```python
from build123d import *

# Parameters (mm, degrees)
F2_R = 9
F3_R = 5


with BuildPart() as f1:
    # F0 (on Front) → F1 (revolve)
    with BuildSketch(Plane.XZ):
        with BuildLine():
            Line((0, 4.25), (0, 0))
            Line((0, 0), (64, 0))
            Line((64, 0), (64, 9))
            Line((64, 9), (20.85148, 9))
            ThreePointArc((20.85148, 9), (13.607068, 7.913606), (7, 4.75))
            Line((7, 4.75), (1.936492, 4.75))
            Line((1.936492, 4.75), (0, 4.25))
        make_face()
    revolve(axis=Axis((32, 0, 0), (1, 0, 0)))

    # F2
    f2_edges = [f1.edges().sort_by_distance(p)[0] for p in [
        (64, 0, -9),
    ]]
    fillet(f2_edges, radius=F2_R)

    # F3
    f3_edges = [f1.edges().sort_by_distance(p)[0] for p in [
        (7, 0, -4.75),
    ]]
    fillet(f3_edges, radius=F3_R)


solid = f1.part
```
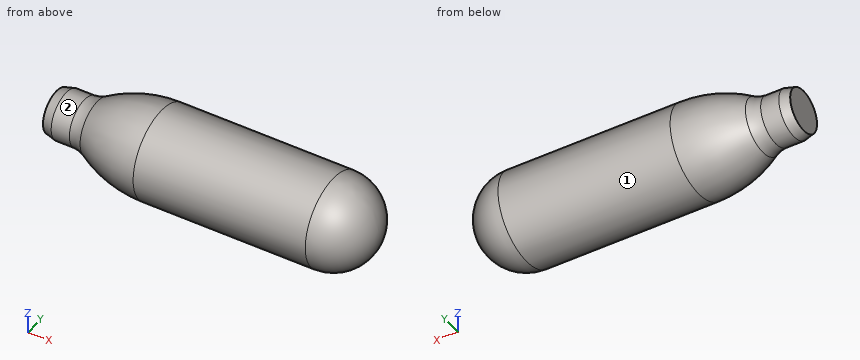
Geometry check sheet. Reference: the model listing, model coordinates, mm. Face numbers are marked on the shaded views. A direction names the side the tool comes from. Give positions to 0.01 mm unless a question says otherwise; leave off trailing zeros. Order: outer loops, then holes, each group sorted by start corner. A loop starts at its lowest first (then second) coordinate and runs counter-clockwise, first axis right, second up.
1. Thickness scan on L1, parallel to X at y = -5.25, z = 3; L2, parallel to Z at x = 58.5, y = -7; L3, parallel to Z at x = 43, y = -5.25. Record the ranges inside material, lowest first.
2. Section check A-A, the plane x = 37.5. Enter the section's corners in (y, z).
3. Access from +Z, -Z, +X, -X, +Y, -Y to the whole of each face (thin tool, end or side, straight path). Record for the marked faces 1 and 2.
4. Section check B-B, the plane x = 59. Enter the section's corners in (y, z), and give its area (3 significant figures).
5. Gauge pin test, flat ends, axial feed: pin 1 Ø1.5 at (x, y) = (42.5, -1.5) entering from -Z; pin 2 Ø5 at (x, y) = (6.5, 6) entering from +Z; pin 3 Ø4 at (x, y) = (42.5, 3.5) entering from +Z. Record the tip position at first contact, or that the pin passes through.
Values follow:
1. L1: x = 9.14 to 61.67
1. L2: z = -4.44 to 4.44
1. L3: z = -7.31 to 7.31
2. outline: circle Ø18 at (0, 0)
3. face 1: +X, -X
3. face 2: -X
4. outline: circle Ø16.12 at (0, 0)
4. area: 204 mm2
5. pin 1: stops at z = -8.97
5. pin 2: stops at z = 3.62
5. pin 3: stops at z = 8.87
